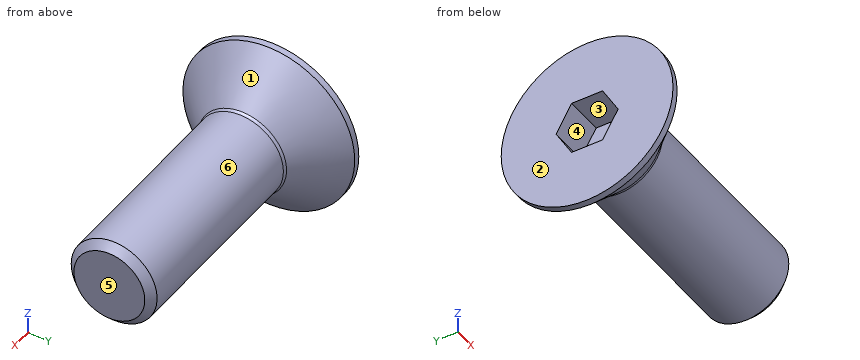
Autodesk Inventor part; units mm, degrees
ref_plane "MSC_PF1" through (0, 0, 0) normal (1, 0, 0) x (0, 1, 0)
ref_plane "MSC_PT1" through (0, 0, 0) normal (1, 0, 0) x (0, 1, 0)
ref_plane "YZ Plane" through (0, 0, 0) normal (1, 0, 0) x (0, 1, 0)
sketch "Skizze1" plane through (0, 0, 0) normal (0, 1, 0) x (-1, 0, 0)
  point P0 (0, 0)
sketch "Skizze2" plane through (0, 0, 0) normal (0, 0, 1) x (-1, 0, 0)
  line L0 (-12, 2) -> (-12, 0)
  line L1 (-2.3, 2) -> (-12, 2)
  line L2 (-0.3, 4) -> (-2.3, 2)
  line L3 (0, 4) -> (-0.3, 4)
  line L4 (0, 0) -> (0, 4)
  line L5 (-12, 0) -> (0, 0)
  line L6 (-12, 0) -> (0, 0)
  line L7 (0, -9.6) -> (0, 1.6)
  line L8 (2.4, 0) -> (-14.4, 0)
  dimension "ParC" = 0.3
  dimension "d43" = 45
  dimension "d44" = 4
  dimension "d45" = 2
  dimension "d46" = 12
  dimension "d47" = 0
  dimension "d48" = 0
revolve "Drehung1" add sketch "Skizze2" angle 360 about axis through (12, 0, 0) along (1, 0, 0)
sketch "Skizze3" plane through (0, 0, 0) normal (-1, 0, 0) x (0, 0, 1)
  line L0 (-1.25, 0.7217) -> (-1.25, -0.7217)
  line L1 (0, 1.4434) -> (-1.25, 0.7217)
  line L2 (1.25, 0.7217) -> (0, 1.4434)
  line L3 (1.25, -0.7217) -> (1.25, 0.7217)
  line L4 (0, -1.4434) -> (1.25, -0.7217)
  line L5 (-1.25, -0.7217) -> (0, -1.4434)
  circle A0 centre (0, 0) radius 1.25 construction
  circle A1 centre (0, 0) radius 2 construction
  dimension "d11" = 2.5
  dimension "d13" = 120
  dimension "d15" = 120
extrude "Extrusion1" cut sketch "Skizze3" against normal blind 1.8
fillet "Rundung1" radius 0.2 1 edges at (2.3, 2, 0)
chamfer "Fase1" distance 0.35 angle 45 1 edges at (12, 2, 0) measured on face at (8.7943, 0.9288, -1.7713)
thread "Gewinde1"
ref_plane "MSC_PF1" through (0, 0, 0) normal (1, 0, 0) x (0, 1, 0)
ref_plane "MSC_PT1" through (0, 0, 0) normal (1, 0, 0) x (0, 1, 0)
equation "\"d43\" = 0.5 * ang"
equation "\"d44\" = 0.5 * dk"
equation "\"d45\" = 0.5 * NND"
equation "\"d46\" = NLG"
equation "\"d11\" = ParS"
equation "\"d16\" = ParT"
equation "\"d18\" = r"
equation "\"d19\" = 0.5 * PTC"
equation "\"d39\" = 0.5 * PTC"
equation "\"NND\" = 4"
equation "\"PTC\" = 0.7"
equation "\"dk\" = 8"
equation "\"ParK\" = 2.3"
equation "\"ParS\" = 2.5"
equation "\"ParT\" = 1.8"
equation "\"r\" = 0.2"
equation "\"NLG\" = 12"
equation "\"ang\" = 90deg"
equation "\"THREADDIA\" = NND"
properties part number "ISO 10642 - M4 x  12" material "Stahl"
Could you check a few things on this model? Use its own coordinates, in mm. Face numbers are marked on the shaded views. A direction names the side the tool comes from. Round coordinates to 2 decimals unless told otherwise and drop trailing zeros. Write each loop counter-clockwise with the first axis right and the second up, starting at its lowest first coordinate (ties: lowest second). Pieces come first, ordered by that corner, then holes.
(1) For pin 1 (2 mm diameter, centred on x = 9, y = -1, fed in from +Z), with a flat end and sliding along its axis, tell me the tip position at first contact or that it passes through.
Findings below:
pin 1: stops at z = 2
(2) Which directions (+Z, -Z, +X, -X, +Y, -Y) give clear straight access to the entire face, cutting with the end or side of a thin tool? Please do the marked faces 4, 5 and 6.
Findings below:
face 4: -X
face 5: +Z, -Z, +X, +Y, -Y
face 6: +X
(3) Suppose I cut it at A-A on x = 9.5. Write out the boundary of the cut face in (y, z).
Findings below:
outline: circle Ø4 at (0, 0)
(4) If I drill on probe 1 along X at (y, z) = (-2.5, 0); probe 2 along X at (y, z) = (-3.5, -0.75); probe 3 along Y at (x, z) = (10.5, 0), over which ranges is the centre line in solid material (lowest first)?
Findings below:
probe 1: x = 0 to 1.8
probe 2: x = 0 to 0.72
probe 3: y = -2 to 2
(5) Thinking about a two-plate mould opening in Y: for the marked faces 1, 2 and 3, which applies, +Y half, -Y half, draft (parallel to the pull), parting line (faces both ways), or undercut?
Findings below:
face 1: parting line
face 2: draft
face 3: undercut
